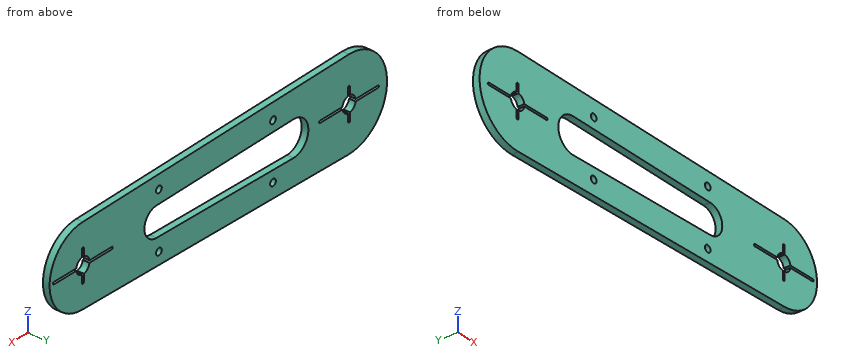
```python
from build123d import *

# Parameters (mm, degrees)
BOSS_EXTRUDE1_DEPTH = 3
SKETCH2_R           = 3.4
SKETCH2_R_2         = 3.375
CUT_EXTRUDE1_DEPTH  = 159.793104384
CUT_EXTRUDE3_DEPTH  = 159.793104384
CUT_EXTRUDE4_DEPTH  = 159.793104384
CUT_EXTRUDE5_DEPTH  = 159.793104384
SKETCH8_R           = 3.5
CUT_EXTRUDE6_DEPTH  = 159.793104384
SKETCH10_R          = 1.5
CUT_EXTRUDE7_DEPTH  = 10


with BuildPart() as part:
    # Sketch1 → Boss-Extrude1 (new body)
    with BuildSketch(Plane(origin=(0, 0, 0), x_dir=(1, 0, 0), z_dir=(0, 1, 0))):
        with BuildLine():
            Line((140.3125, 17.497209599), (0.357142857, 19.99681097))
            ThreePointArc((0.357142857, 19.99681097), (-19.999202727, 0.178578547), (0, -20))
            Line((0, -20), (140, -17.5))
            ThreePointArc((140, -17.5), (157.499302386, -0.156256229), (140.3125, 17.497209599))
        make_face()
    extrude(amount=BOSS_EXTRUDE1_DEPTH)

    # Sketch2 → Cut-Extrude1 (cut, through all)
    with BuildSketch(Plane(origin=(0, 3, 0), x_dir=(1, 0, 0), z_dir=(0, 1, 0))):
        with Locations(Location((0, 0, 0), (0, 0, 270))):
            Circle(SKETCH2_R)
        with Locations(Location((140, 0, 0), (0, 0, 270))):
            Circle(SKETCH2_R_2)
    extrude(amount=-CUT_EXTRUDE1_DEPTH, mode=Mode.SUBTRACT)

    # Sketch4 → Cut-Extrude3 (cut, through all)
    with BuildSketch(Plane(origin=(0, 3, 0), x_dir=(1, 0, 0), z_dir=(0, 1, 0))):
        with BuildLine():
            ThreePointArc((101.494647455, -6.185682468), (107.64017994, 0.394224207), (101.283865867, 6.770744637))
            Line((101.283865867, 6.770744637), (29.173044697, 8.058643229))
            ThreePointArc((29.173044697, 8.058643229), (21.397292905, 0.29833633), (29.157599804, -7.477415462))
            Line((29.157599804, -7.477415462), (101.052392136, -6.193579885))
            Line((101.052392136, -6.193579885), (101.494647455, -6.185682468))
        make_face()
    extrude(amount=-CUT_EXTRUDE3_DEPTH, mode=Mode.SUBTRACT)

    # Sketch6 → Cut-Extrude4 (cut, through all)
    with BuildSketch(Plane(origin=(0, 0, 0), x_dir=(1, 0, 0), z_dir=(0, 1, 0))):
        with BuildLine():
            Line((-15.22, 0.5), (15.22, 0.5))
            ThreePointArc((15.22, 0.5), (15.72, 0), (15.22, -0.5))
            Line((15.22, -0.5), (-15.22, -0.5))
            ThreePointArc((-15.22, -0.5), (-15.72, 0), (-15.22, 0.5))
        make_face()
        with BuildLine():
            Line((-0.5, -6.855), (-0.5, 6.855))
            ThreePointArc((-0.5, 6.855), (0, 7.355), (0.5, 6.855))
            Line((0.5, 6.855), (0.5, -6.855))
            ThreePointArc((0.5, -6.855), (0, -7.355), (-0.5, -6.855))
        make_face()
    extrude(amount=CUT_EXTRUDE4_DEPTH, mode=Mode.SUBTRACT)

    # Sketch7 → Cut-Extrude5 (cut, through all)
    with BuildSketch(Plane(origin=(0, 3, 0), x_dir=(1, 0, 0), z_dir=(0, 1, 0))):
        with BuildLine():
            Line((155.22, -0.5), (124.78, -0.5))
            ThreePointArc((124.78, -0.5), (124.28, 0), (124.78, 0.5))
            Line((124.78, 0.5), (155.22, 0.5))
            ThreePointArc((155.22, 0.5), (155.72, 0), (155.22, -0.5))
        make_face()
        with BuildLine():
            Line((139.5, -6.855), (139.5, 6.855))
            ThreePointArc((139.5, 6.855), (140, 7.355), (140.5, 6.855))
            Line((140.5, 6.855), (140.5, -6.855))
            ThreePointArc((140.5, -6.855), (140, -7.355), (139.5, -6.855))
        make_face()
    extrude(amount=-CUT_EXTRUDE5_DEPTH, mode=Mode.SUBTRACT)

    # Sketch8 → Cut-Extrude6 (cut, through all)
    with BuildSketch(Plane(origin=(0, 3, 0), x_dir=(1, 0, 0), z_dir=(0, 1, 0))):
        Circle(SKETCH8_R)
        with Locations((140, 0)):
            Circle(SKETCH8_R)
    extrude(amount=-CUT_EXTRUDE6_DEPTH, mode=Mode.SUBTRACT)

    # Sketch10 → Cut-Extrude7 (cut)
    with BuildSketch(Plane(origin=(0, 3, 0), x_dir=(1, 0, 0), z_dir=(0, 1, 0))):
        with Locations(Location((40, 12.866071293, 0), (0, 0, 270))):
            Circle(SKETCH10_R)
        with Locations(Location((40, -12.055388552, 0), (0, 0, 270))):
            Circle(SKETCH10_R)
        with Locations(Location((100, -12.055388552, 0), (0, 0, 270))):
            Circle(SKETCH10_R)
        with Locations(Location((100, 12.866071293, 0), (0, 0, 270))):
            Circle(SKETCH10_R)
    extrude(amount=-CUT_EXTRUDE7_DEPTH, mode=Mode.SUBTRACT)


solid = part.part
```
Check sheet for the modelled part. Datum: model origin and axes. Units: mm. Round coordinates to 2 decimals unless told otherwise and drop trailing zeros. Loops run counter-clockwise (first coordinate to the right, second up) from the corner with the lowest first, then second, coordinate; pieces in that order, holes last. Notation, with made-up numbers: (51.5, 22.5) - (58.5, 22.5) arc R28 cw to (58.5, 51.5) - close; hole circle Ø2 at (-22, 87.5). An arc over 180 degrees is marked (long way). Answer as a JSON object with one key per item and string values. Group by question number.
Q1. Sectioned sample at B-B, the plane y = 2.3. Count the separate pieces of the cut face and the enclosed holes in it, plus the area to 3 significant figures.
Q2. Scan lines: line 1 along X through (y, z) = (1.9, 12); line 2 along X through (y, z) = (1.4, -12.5); line 3 along Z through (x, y) = (100, 1.7). Record each from-to range of solid material in increasing order. Write a range as [from, to].
Q3. Sectioned sample at D-D, the plane x = 113.5. Enter the section's corners in (y, z), plus the area to 3 significant figures.
Q4. Sectioned sample at A-A, the plane x = 25. Enter the section's corners in (y, z), plus the area to 3 significant figures.
Q5. Sectioned sample at C-C, the plane x = 89.5. Enter the section's corners in (y, z), plus the area to 3 significant figures.
Q6. Gauge pin test, flat ends, axial feed: P1, Ø1.5, axis at x = 125.5, y = 2, coming from the +Z side; P2, Ø1.5, axis at x = 133, y = 2, coming from the +Z side; P3, Ø0.9, axis at x = 8, y = 2, coming from the +Z side. Record the tip position at first contact, or that the pin passes through.
Solution:
{
 "1": {"separate pieces": "1", "enclosed holes": "7", "area": "5,000 mm²"},
 "2": {"line 1": "x = [-16, 38.5], [41.5, 98.5], [101.5, 152.74]", "line 2": "x = [-15.61, 38.55], [41.45, 98.55], [101.45, 152.25]", "line 3": "z = [-18.22, -14.37], [-11.37, -6.79], [6.21, 10.56], [13.56, 18.21]"},
 "3": {"outline": "(0, -17.98) - (3, -17.98) - (3, 17.97) - (0, 17.97) - close", "area": "108 mm²"},
 "4": {"outline": "(0, -19.56) - (3, -19.56) - (3, -6.85) - (0, -6.85) - close; (0, 6.27) - (3, 6.27) - (3, 19.55) - (0, 19.55) - close", "area": "78.0 mm²"},
 "5": {"outline": "(0, -18.4) - (3, -18.4) - (3, -6.98) - (0, -6.98) - close; (0, 6.4) - (3, 6.4) - (3, 18.4) - (0, 18.4) - close", "area": "70.3 mm²"},
 "6": {"P1": "stops at z = 17.77", "P2": "stops at z = 17.64", "P3": "stops at z = 19.87"}
}
